Here's how the part is built. I have some questions about the finished solid (model axes, mm). Face numbers are marked on the shaded views. A direction names the side the tool comes from. Give positions to 0.01 mm unless a question says otherwise; leave off trailing zeros. Loops run counter-clockwise (first coordinate to the right, second up) from the corner with the lowest first, then second, coordinate; pieces in that order, holes last.
Q1. Suppose I cut it at B-B (x = 0). List the corners of the cut face in (y, z) for me, and give its area (3 significant figures).
Q2. Thinking about a two-plate mould opening in Y: for the marked faces 1, 2 and 3, which applies, pulls with the +Y half, pulls with the -Y half, needs draft (parallel to the pull), parting line crosses it, or undercut?
Q3. Suppose I cut it at A-A (y = 0). List the corners of the cut face in (x, z) for me, and give its area (3 significant figures).
Q4. For the marked faces 4, 5, 6 and 7, which set-ups out of +Z, -Z, +X, -X, +Y, -Y let a thin tool reach every point of the face, with its end or its side?
Q5. I need wall thicknesses on probe 1 along Y at (x, z) = (0, -2.5); probe 2 along X at (y, z) = (-16, -4.5) (1 decimal); probe 3 along X at (y, z) = (-7.5, 7.25). Which ranges of each line are inside material? Lowest first, please.
Q6. I'm going to push flat-ended pins straight in: P1, Ø1.9, axis at y = -16.5, z = -3.5, coming from the +X side; P2, Ø1, axis at x = 15, y = -8, coming from the -Z side; P3, Ø8, axis at x = 12.5, z = -3, coming from the +Y side. Where does each tip first touch, or does it pass through?
Q7. Suppose I cut it at C-C (z = -4). Count the separate pieces of the cut face and the enclosed holes in it, and give its area (3 significant figures).
Q8. Suppose I cut it at D-D (x = -14.5). List the corners of the cut face in (y, z) for me.
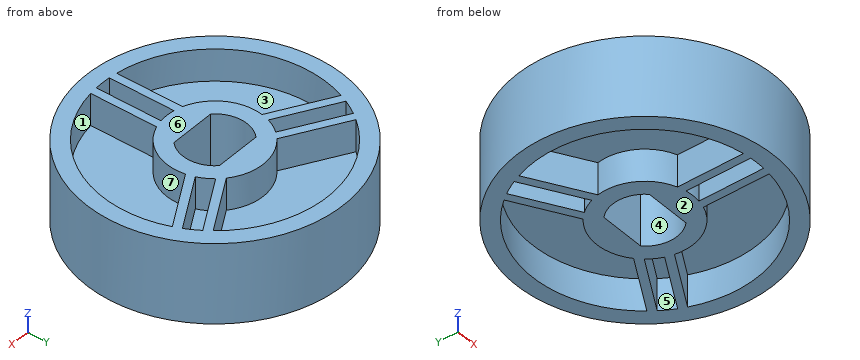
Autodesk Inventor part; units mm, degrees
ref_plane "YZ Plane" through (0, 0, 0) normal (1, 0, 0) x (0, 1, 0)
ref_plane "XZ Plane" through (0, 0, 0) normal (0, 1, 0) x (-1, 0, 0)
ref_plane "XY Plane" through (0, 0, 0) normal (0, 0, 1) x (1, 0, 0)
sketch "Sketch1" plane through (0, 0, 0) normal (0, 0, 1) x (1, 0, 0)
  line L0 (-4.4901, 4.4901) -> (4.4901, 4.4901)
  line L1 (4.4901, 4.4901) -> (4.4901, -4.4901) construction
  line L2 (4.4901, -4.4901) -> (-4.4901, -4.4901)
  line L3 (-4.4901, -4.4901) -> (-4.4901, 4.4901) construction
  arc A0 (-4.4901, 4.4901) -> (-4.4901, -4.4901) centre (0, 0) ccw
  arc A1 (4.4901, -4.4901) -> (4.4901, 4.4901) centre (0, 0) ccw
  arc A2 (6.1896, 7.2398) -> (9.3646, 1.7405) centre (0, 0) ccw
  arc A3 (17.4625, 13.7482) -> (20.6375, 8.2489) centre (0, 0) ccw
  circle A4 centre (0, 0) radius 25.4
  line L4 (6.1896, 7.2398) -> (17.4625, 13.7482)
  line L5 (7.3398, 6.0707) -> (18.4045, 12.4589)
  line L6 (19.992, 9.7093) -> (8.9273, 3.3211)
  line L7 (9.3646, 1.7405) -> (20.6375, 8.2489)
  line L8 (0, 0) -> (19.2474, 11.1125) construction
  arc A5 (7.3398, 6.0707) -> (6.1896, 7.2398) centre (0, 0) ccw
  arc A6 (8.9273, 3.3211) -> (7.3398, 6.0707) centre (0, 0) ccw
  arc A7 (9.3646, 1.7405) -> (8.9273, 3.3211) centre (0, 0) ccw
  arc A8 (18.4045, 12.4589) -> (17.4625, 13.7482) centre (0, 0) ccw
  arc A9 (19.992, 9.7093) -> (18.4045, 12.4589) centre (0, 0) ccw
  arc A10 (20.6375, 8.2489) -> (19.992, 9.7093) centre (0, 0) ccw
  line L9 (-9.3646, 1.7405) -> (-20.6375, 8.2489)
  line L10 (-8.9273, 3.3211) -> (-19.992, 9.7093)
  line L11 (-18.4045, 12.4589) -> (-7.3398, 6.0707)
  line L12 (-6.1896, 7.2398) -> (-17.4625, 13.7482)
  arc A11 (-8.9273, 3.3211) -> (-9.3646, 1.7405) centre (0, 0) ccw
  arc A12 (-6.1896, 7.2398) -> (-7.3398, 6.0707) centre (0, 0) ccw
  arc A13 (-19.992, 9.7093) -> (-20.6375, 8.2489) centre (0, 0) ccw
  arc A14 (-17.4625, 13.7482) -> (-18.4045, 12.4589) centre (0, 0) ccw
  line L13 (3.175, -8.9803) -> (3.175, -21.997)
  line L14 (1.5875, -9.3918) -> (1.5875, -22.1682)
  line L15 (-1.5875, -22.1682) -> (-1.5875, -9.3918)
  line L16 (-3.175, -8.9803) -> (-3.175, -21.997)
  arc A15 (1.5875, -9.3918) -> (3.175, -8.9803) centre (0, 0) ccw
  arc A16 (-3.175, -8.9803) -> (-1.5875, -9.3918) centre (0, 0) ccw
  arc A17 (1.5875, -22.1682) -> (3.175, -21.997) centre (0, 0) ccw
  arc A18 (-3.175, -21.997) -> (-1.5875, -22.1682) centre (0, 0) ccw
  dimension "d4" = 6.35
  dimension "d5" = 8.9803
  dimension "d6" = 8.9803
  dimension "d7" = 19.05
  dimension "d8" = 44.45
  dimension "d9" = 50.8
  dimension "d14" = 1.5875
  dimension "d15" = 3.175
  dimension "d16" = 1.5875
  dimension "d17" = 1.5875
  dimension "d18" = 30
  dimension "d21" = 360
extrude "Extrusion1" add sketch "Sketch1" along normal mid plane 15.875 contours A5 A6 A7 A2 | L4 A8 L5 A5 | A2 L11 A3 L12 | L6 A10 L7 A7 | A2 L9 A3 L10 | L13 A3 L14 A2 | A2 L15 A3 L16 | A4
extrude "Extrusion2" add sketch "Sketch1" along normal mid plane 3.175 contours A5 A6 A7 A2 | A2 L12 A3 L4 | A2 L11 A3 L12 | L5 A9 L6 A6 | A2 L10 A3 L11 | A2 L9 A3 L10 | L7 A3 L13 A2 | A2 L16 A3 L9 | L13 A3 L14 A2 | A2 L15 A3 L16 | L14 A3 L15 A2
equation "\"d5\" = d6"
equation "\"d16\" = d14"
equation "\"d17\" = 0.5 * d15"
properties part number "blue wheel hub"
Solutions:
1. outline: (-25.4, -7.94) - (-22.22, -7.94) - (-22.22, -1.59) - (-9.52, -1.59) - (-9.52, -7.94) - (-4.49, -7.94) - (-4.49, 7.94) - (-9.52, 7.94) - (-9.52, 1.59) - (-22.22, 1.59) - (-22.22, 7.94) - (-25.4, 7.94) - close; (4.49, -7.94) - (9.53, -7.94) - (9.53, -1.59) - (22.23, -1.59) - (22.23, -7.94) - (25.4, -7.94) - (25.4, 7.94) - (22.23, 7.94) - (22.23, 1.59) - (9.53, 1.59) - (9.53, 7.94) - (4.49, 7.94) - close
1. area: 341 mm2
2. face 1: undercut
2. face 2: needs draft
2. face 3: undercut
3. outline: (-25.4, -7.94) - (-22.23, -7.94) - (-22.23, -1.59) - (-9.53, -1.59) - (-9.53, -7.94) - (-6.35, -7.94) - (-6.35, 7.94) - (-9.53, 7.94) - (-9.53, 1.59) - (-22.23, 1.59) - (-22.23, 7.94) - (-25.4, 7.94) - close; (6.35, -7.94) - (9.52, -7.94) - (9.52, -1.59) - (22.22, -1.59) - (22.22, -7.94) - (25.4, -7.94) - (25.4, 7.94) - (22.22, 7.94) - (22.22, 1.59) - (9.52, 1.59) - (9.52, 7.94) - (6.35, 7.94) - close
3. area: 282 mm2
4. face 4: +Z, -Z
4. face 5: -Z
4. face 6: +Z, +X, -X, +Y, -Y
4. face 7: +Z
5. probe 1: y = -25.4 to -22.22, -9.52 to -4.49, 4.49 to 9.53, 22.23 to 25.4
5. probe 2: x = -19.7 to -15.4, -3.2 to -1.6, 1.6 to 3.2, 15.4 to 19.7
5. probe 3: x = -24.27 to -20.92, -5.87 to 5.87, 20.92 to 24.27
6. P1: stops at x = 20.08
6. P2: stops at z = -1.59
6. P3: stops at y = 23.94
7. separate pieces: 1
7. enclosed holes: 7
7. area: 779 mm2
8. outline: (-20.85, -7.94) - (-16.84, -7.94) - (-16.84, -1.59) - (4.71, -1.59) - (4.71, -7.94) - (6.54, -7.94) - (6.54, -1.59) - (10.2, -1.59) - (10.2, -7.94) - (12.04, -7.94) - (12.04, -1.59) - (16.84, -1.59) - (16.84, -7.94) - (20.85, -7.94) - (20.85, 7.94) - (16.84, 7.94) - (16.84, 1.59) - (12.04, 1.59) - (12.04, 7.94) - (10.2, 7.94) - (10.2, 1.59) - (6.54, 1.59) - (6.54, 7.94) - (4.71, 7.94) - (4.71, 1.59) - (-16.84, 1.59) - (-16.84, 7.94) - (-20.85, 7.94) - close
